Part model, mm, in its own coordinate system. A direction names the side the tool comes from. Coordinates: 2 decimals unless noted, no trailing zeros. Write each question's results on one line, items separated by ' | '.
from build123d import *

# Parameters (mm, degrees)
SKETCH_R        = 8.5
PAD001_DEPTH    = 6
CHAMFER_ANGLE   = 55
CHAMFER_SIZE    = 3.5
SKETCH007_R     = 3.5
POCKET_DEPTH    = 20.5
SKETCH5_R       = 6.35
POCKET001_DEPTH = 3
SKETCH6_R       = 3.1
POCKET002_DEPTH = 6.1


with BuildPart() as part:
    # Sketch → Pad001 (new body)
    with BuildSketch(Plane.XY):
        Circle(SKETCH_R)
    extrude(amount=PAD001_DEPTH)

    # Chamfer
    chamfer_edges = [part.edges().sort_by_distance(p)[0] for p in [
        (-8.5, 0, 6),
    ]]
    chamfer_side = part.faces().sort_by_distance((-8.5, 0, 3))[0]
    chamfer(chamfer_edges, length=CHAMFER_SIZE, angle=CHAMFER_ANGLE, reference=chamfer_side)

    # Sketch1 → AdditiveLoft section 0
    with BuildSketch(Plane.XY):
        Polygon((-2.104759, 5.081337), (0, 8), (2.104759, 5.081337), (5.656854, 5.656854), (5.081337, 2.104759), (8, 0), (5.081337, -2.104759), (5.656854, -5.656854), (2.104759, -5.081337), (0, -8), (-2.104759, -5.081337), (-5.656854, -5.656854), (-5.081337, -2.104759), (-8, 0), (-5.081337, 2.104759), (-5.656854, 5.656854), align=None)
    # Sketch007 → AdditiveLoft section 1
    with BuildSketch(Plane.XY.offset(22.5)):
        Circle(SKETCH007_R)
    loft()

    # Sketch3 → Pocket (cut)
    with BuildSketch(Plane(origin=(0, 0, 0), x_dir=(-1, 0, 0), z_dir=(0, 0, -1))):
        with BuildLine():
            ThreePointArc((2.592296, -1.7), (0, 3.1), (-2.592296, -1.7))
            Line((2.592296, -1.7), (-2.592296, -1.7))
        make_face()
    extrude(amount=-POCKET_DEPTH, mode=Mode.SUBTRACT)

    # Sketch5 → Pocket001 (cut)
    with BuildSketch(Plane(origin=(0, 0, 0), x_dir=(-1, 0, 0), z_dir=(0, 0, -1))):
        Circle(SKETCH5_R)
    extrude(amount=-POCKET001_DEPTH, mode=Mode.SUBTRACT)

    # Sketch6 → Pocket002 (cut)
    with BuildSketch(Plane(origin=(0, 0, 3), x_dir=(-1, 0, 0), z_dir=(0, 0, -1))):
        Circle(SKETCH6_R)
    extrude(amount=-POCKET002_DEPTH, mode=Mode.SUBTRACT)


solid = part.part
(1) Two-plate mould, pull along Y, no slides. Class faces 1 (the flat face through (0, 1, 20.5)), 2 (the cylindrical face through (4.57, 7.167, 1.232)), 3 (the flat face through (0, 0, 22.5)): released by +Y, released by -Y, zero draft, split by the parting line, or undercut.
Return value:
face 1: undercut | face 2: split by the parting line | face 3: zero draft
(2) Flat gauge pins, fed straight in: P1, Ø2, axis at y = -4.5, z = 14, coming from the +X side; P2, Ø4, axis at x = 2.5, y = -1, coming from the -Z side; P3, Ø4, axis at y = 4, z = 5.5, coming from the -X side; P4, Ø4, axis at x = -4, y = 0.5, coming from the +Z side. Where does each tip first touch, or does it go through?
Return value:
P1: stops at x = 3.77 | P2: stops at z = 3 | P3: stops at x = -6.05 | P4: stops at z = 22.5
(3) 3-axis set-ups, long thin cutter, end or side, ignore diameter. For faces 4 (the conical face through (4.83, -2, 4.79)), 5 (the flat face through (-3, 2, 3)): which of +Z, -Z, +X, -X, +Y, -Y reach the whole face in a straight line?
Return value:
face 4: +Z | face 5: -Z
(4) Wall check: line 1 (Y direction, x = 0, z = 1.95); line 2 (X direction, y = 2, z = 13); line 3 (X direction, y = -2.5, z = 5.75). Give the ranges that are in metal, low to high. Write a range as from..to.
Return value:
line 1: y = -8.5..-6.35, 6.35..8.5 | line 2: x = -4..-2.37, 2.37..4 | line 3: x = -4.67..-1.83, 1.83..4.67
